The listing builds one solid part. Answer for the finished solid, in the listing's coordinates (mm). A direction names the side the tool comes from. Coordinates: 2 decimals unless noted, no trailing zeros. Order: outer loops, then holes, each group sorted by start corner. A loop starts at its lowest first (then second) coordinate and runs counter-clockwise, first axis right, second up. Notation, with made-up numbers: (-1.75, 75.25) - (5.25, 75.25) arc R10 ccw to (5.25, 91.25) - close; hole circle Ø10 at (8, 80). An arc over 180 degrees is marked (long way). Use a Markdown table: item, result. Add a question column.
Item 1: The part is cut by section C-C, the plane z = -25.85. Give the vertices of the cut face in (x, y).
Item 2: The part is cut by section A-A, the plane x = -5. Give the vertices of the cut face in (y, z), then the cut area to 3 significant figures.
Item 3: The mould has two halves that part along Z. Classify faces 1 (the cylindrical face through (-9.74, 1.972, -93.683)), 2 (the flat face through (3, -9, -87.35)), 3 (the flat face through (-5, 0, -45)): released by +Z, released by -Z, zero draft, split by the parting line, or undercut.
Item 4: For faces 4 (the cylindrical face through (-5.69, 1.97, -74.52)), 5 (the flat face through (4, -9, -4.35)), 6 (the flat face through (2, -9, -45)), determine the directions among +Z, -Z, +X, -X, +Y, -Y from which every point of the face is accessible in a straight line to the end or side of a thin tool.
Item 5: The part is cut by section B-B, the plane y = 1.5. State how many separate pieces and enclosed holes the cut face has, then the cut area to 3 significant figures.
Item 6: Flat-ended cylindrical pins translate along their axes: P1, Ø3, axis at x = 0, z = 0, coming from the -Y side; P2, Ø10, axis at x = 0, y = -13.5, coming from the +Z side; P3, Ø4, axis at x = -5, z = -65.85, coming from the -Y side; P4, Ø8, axis at x = -1, y = -15.5, coming from the -Z side. Find the tip coordinate at first contact, or state that the pin passes through.
Item 7: Find the intervals of material crossed by line 1 along Z through (x, y) = (0, 1.85); line 2 along Z through (x, y) = (-5, 1.5); line 3 along X through (y, z) = (2.3, -91.7), in increasing order.
Item 8: The part is cut by section D-D, the plane z = -91.7. Give the vertices of the cut face in (x, y).
Autodesk Inventor part; units mm, degrees
ref_plane "YZ Plane" through (0, 0, 0) normal (1, 0, 0) x (0, 1, 0)
ref_plane "XZ Plane" through (0, 0, 0) normal (0, 1, 0) x (-1, 0, 0)
ref_plane "XY Plane" through (0, 0, 0) normal (0, 0, 1) x (1, 0, 0)
sketch "Sketch1" plane through (0, 0, 0) normal (0, 1, 0) x (-1, 0, 0)
  line L0 (0, 0) -> (10, 0)
  line L1 (10, 0) -> (10, -91.7)
  line L2 (10, -91.7) -> (0, -91.7)
  line L3 (0, -91.7) -> (0, 0)
  circle A0 centre (10, 0) radius 2
  circle A1 centre (0, 0) radius 2
  circle A2 centre (10, -91.7) radius 2
  circle A3 centre (0, -91.7) radius 2
  line L4 (10, 0) -> (15, 0)
  line L5 (15, 0) -> (15, 4)
  line L6 (15, 4) -> (10, 4)
  line L7 (10, 4) -> (10, 0)
  line L8 (0, -91.7) -> (-5, -91.7)
  line L9 (-5, -91.7) -> (-5, -95.7)
  line L10 (-5, -95.7) -> (0, -95.7)
  line L11 (0, -95.7) -> (0, -91.7)
  line L12 (15, 4) -> (-5, 4)
  line L13 (-5, 4) -> (-5, -95.7)
  line L14 (-5, -95.7) -> (15, -95.7)
  line L15 (15, -95.7) -> (15, 4)
  line L16 (5, 0) -> (5, -91.7)
  line L17 (5, -20.85) -> (5, -70.85)
  line L18 (5, -15.85) -> (5, -25.85)
  line L19 (5, -65.85) -> (5, -75.85)
  circle A4 centre (5, -15.85) radius 1.5
  circle A5 centre (5, -25.85) radius 1.5
  circle A6 centre (5, -65.85) radius 1.5
  circle A7 centre (5, -75.85) radius 1.5
  point P0 (5, -45.85)
  point P1 (-2, -91.7)
  point P2 (0, -93.7)
  dimension "d0" = 10
  dimension "d1" = 91.7
  dimension "d2" = 4
  dimension "d3" = 4
  dimension "d4" = 4
  dimension "d5" = 4
  dimension "d6" = 5
  dimension "d7" = 4
  dimension "d8" = 5
  dimension "d9" = 4
  dimension "d10" = 50
  dimension "d11" = 10
  dimension "d12" = 10
  dimension "d13" = 3
  dimension "d14" = 3
  dimension "d15" = 3
  dimension "d16" = 3
extrude "Extrusion1" add sketch "Sketch1" along normal blind 4 contours A1 L3 A3 L8 L13 L12 L7 A0 L0 | L0 L16 A4 A5 A6 A7 L2 A3 L3 A1 | L0 A0 L1 A2 L2 L16 A7 A6 A5 A4 | L2 A2 L1 A0 L4 L15 L14 L11 A3 | A3 L11 L10 L9 L8 | L7 L6 L5 L4 A0
sketch "Sketch2" plane through (0, 0, 0) normal (0, -1, 0) x (1, 0, 0)
  line L0 (5, 4) -> (5, -95.7)
  line L1 (5, -87.35) -> (5, -4.35)
  line L2 (5, -4.35) -> (2, -4.35)
  line L3 (2, -4.35) -> (2, -87.35)
  line L4 (2, -87.35) -> (5, -87.35)
  line L5 (5, -87.35) -> (5, -4.35)
  point P0 (0, 0)
  point P1 (5, -45.85)
  dimension "d19" = 83
  dimension "d20" = 3
extrude "Extrusion2" add sketch "Sketch2" along normal blind 18
properties part number "side_wall1"
Solution:
| question | item | result |
|---|---|---|
| 1 | outline | (-15, 0) - (-6.5, 0) - (-6.5, 4) - (-15, 4) - close; (-3.5, 0) - (2, 0) - (2, -18) - (5, -18) - (5, 4) - (-3.5, 4) - close |
| 2 | outline | (0, -95.7) - (4, -95.7) - (4, -77.35) - (0, -77.35) - close; (0, -74.35) - (4, -74.35) - (4, -67.35) - (0, -67.35) - close; (0, -64.35) - (4, -64.35) - (4, -27.35) - (0, -27.35) - close; (0, -24.35) - (4, -24.35) - (4, -17.35) - (0, -17.35) - close; (0, -14.35) - (4, -14.35) - (4, 4) - (0, 4) - close |
| 2 | area | 351 mm2 |
| 3 | face 1 | undercut |
| 3 | face 2 | released by -Z |
| 3 | face 3 | zero draft |
| 4 | face 4 | +Y, -Y |
| 4 | face 5 | +Z, +X, -X, -Y |
| 4 | face 6 | +Z, -Z, -X, -Y |
| 5 | separate pieces | 1 |
| 5 | enclosed holes | 8 |
| 5 | area | 1,920 mm2 |
| 6 | P1 | passes through |
| 6 | P2 | stops at z = -4.35 |
| 6 | P3 | stops at y = 0 |
| 6 | P4 | stops at z = -87.35 |
| 7 | line 1 | z = -95.7 to -93.7, -89.7 to -2, 2 to 4 |
| 7 | line 2 | z = -95.7 to -77.35, -74.35 to -67.35, -64.35 to -27.35, -24.35 to -17.35, -14.35 to 4 |
| 7 | line 3 | x = -15 to -12, -8 to -2, 2 to 5 |
| 8 | outline | (-15, 0) - (-12, 0) - (-12, 4) - (-15, 4) - close; (-8, 0) - (-2, 0) - (-2, 4) - (-8, 4) - close; (2, 0) - (5, 0) - (5, 4) - (2, 4) - close |
